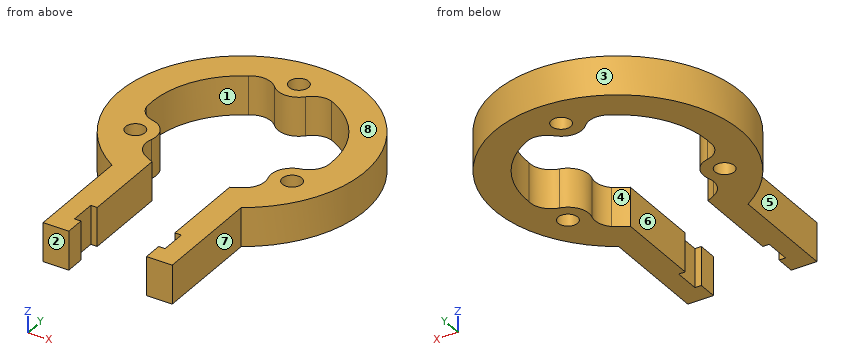
```python
from build123d import *

# Parameters (mm, degrees)
ESQUISSE1_R        = 1.5
BOSS_EXTRU_2_DEPTH = 6


with BuildPart() as part:
    # Esquisse1 → Boss.-Extru.2 (new body)
    with BuildSketch(Plane.XY):
        with BuildLine():
            Line((-6, -33.155494421), (-6, -30.155494421))
            Line((-6, -30.155494421), (-7, -30.155494421))
            Line((-7, -30.155494421), (-7, -26.155494421))
            Line((-7, -26.155494421), (-6, -26.155494421))
            Line((-6, -26.155494421), (-6, -12.649110641))
            ThreePointArc((-6, -12.649110641), (-6.653410863, -12.317959405), (-7.288606081, -11.953084179))
            ThreePointArc((-7.288606081, -11.953084179), (-8.912631465, -10.307392628), (-9.031496673, -7.998360322))
            ThreePointArc((-9.031496673, -7.998360322), (-9.309773091, -5.375), (-11.442531564, -3.822325392))
            ThreePointArc((-11.442531564, -3.822325392), (-13.054716827, -2.946828253), (-13.935938611, -1.337764944))
            ThreePointArc((-13.935938611, -1.337764944), (-12.367555464, 6.560760004), (-6.707371512, 12.288660114))
            ThreePointArc((-6.707371512, 12.288660114), (-4.47014813, 12.872261577), (-2.411034891, 11.820685714))
            ThreePointArc((-2.411034891, 11.820685714), (0, 10.75), (2.411034891, 11.820685714))
            ThreePointArc((2.411034891, 11.820685714), (3.975330286, 12.779130538), (5.80943088, 12.737759334))
            ThreePointArc((5.80943088, 12.737759334), (11.865562564, 7.430237213), (13.995977593, -0.335575935))
            ThreePointArc((13.995977593, -0.335575935), (13.382779595, -2.564868949), (11.442531564, -3.822325392))
            ThreePointArc((11.442531564, -3.822325392), (9.309773091, -5.375), (9.031496673, -7.998360322))
            ThreePointArc((9.031496673, -7.998360322), (9.079386541, -9.832302285), (8.126507731, -11.399994391))
            ThreePointArc((8.126507731, -11.399994391), (7.090812931, -12.071469338), (6, -12.649110641))
            Line((6, -12.649110641), (6, -26.155494421))
            Line((6, -26.155494421), (7, -26.155494421))
            Line((7, -26.155494421), (7, -30.155494421))
            Line((7, -30.155494421), (6, -30.155494421))
            Line((6, -30.155494421), (6, -33.155494421))
            Line((6, -33.155494421), (10, -33.155494421))
            Line((10, -33.155494421), (10, -16.155494421))
            ThreePointArc((10, -16.155494421), (0, 19), (-10, -16.155494421))
            Line((-10, -16.155494421), (-10, -33.155494421))
            Line((-10, -33.155494421), (-6, -33.155494421))
        make_face()
        with Locations((0, 14)):
            Circle(ESQUISSE1_R, mode=Mode.SUBTRACT)
        with Locations((12.124355653, -7)):
            Circle(ESQUISSE1_R, mode=Mode.SUBTRACT)
        with Locations((-12.124355653, -7)):
            Circle(ESQUISSE1_R, mode=Mode.SUBTRACT)
    extrude(amount=BOSS_EXTRU_2_DEPTH)


solid = part.part
```
The listing builds one solid part. Answer for the finished solid, in the listing's coordinates (mm). Face numbers are marked on the shaded views. A direction names the side the tool comes from. Coordinates: 2 decimals unless noted, no trailing zeros. Write each loop counter-clockwise with the first axis right and the second up, starting at its lowest first coordinate (ties: lowest second). Pieces come first, ordered by that corner, then holes. Notation, with made-up numbers: (54.25, 41) - (75.25, 41) arc R11 cw to (75.25, 49) - close; hole circle Ø4 at (2, 53). An arc over 180 degrees is marked (long way). One line per item, written item: value.
1) Each of these flat-tipped pins is pushed along its axis until it touches: pin 1 Ø2 at (x, z) = (-5, 4) entering from +Y; pin 2 Ø1.1 at (x, z) = (6.5, 1.5) entering from +Y; pin 3 Ø3.5 at (x, y) = (12.12, -7) entering from +Z; pin 4 Ø1.5 at (x, z) = (4.5, 1) entering from -Y. Where does it stop, or does it pass through?
Geometry check:
pin 1: stops at y = 18.57
pin 2: stops at y = 18.04
pin 3: stops at z = 6
pin 4: stops at y = 12.71
2) Consider line 1 along X through (y, z) = (-26.5, 2.45); line 2 along X through (y, z) = (-18.5, 5.4); line 3 along Y through (x, z) = (12.5, 5.85). Determine where each line is inside the solid, lowest interval first. Write a range as from..to.
Geometry check:
line 1: x = -10..-7, 7..10
line 2: x = -10..-6, 6..10
line 3: y = -14.31..-8.45, -5.55..-3.39, 6.3..14.31
3) Find section D-D (x = -13). Give the vertices of the cut face in (y, z).
Geometry check:
outline: (-13.86, 0) - (-8.22, 0) - (-8.22, 6) - (-13.86, 6) - close; (-5.78, 0) - (-3, 0) - (-3, 6) - (-5.78, 6) - close; (5.2, 0) - (13.86, 0) - (13.86, 6) - (5.2, 6) - close
4) Find section C-C (z = 3.5). Count the separate pieces of the cut face and the enclosed holes in it, and give its area (3 significant figures).
Geometry check:
separate pieces: 1
enclosed holes: 3
area: 611 mm2
5) For a pull along X with two mould halves and no side action, classify the marked faces 1, 2 and 3 as pulls with the +X half, pulls with the -X half, needs draft (parallel to the pull), parting line crosses it, or undercut.
Geometry check:
face 1: undercut
face 2: needs draft
face 3: parting line crosses it
6) A tool of negligible diameter and unlimited length cuts with its end or side. For the marked faces 4, 5, 6, 7 and 8, from which of +Z, -Z, +X, -X, +Y, -Y can it reach the whole face along a straight path? Write none if from no direction.
Geometry check:
face 4: +Z, -Z
face 5: +Z, -Z, -X, -Y
face 6: +Z, -Z, -Y
face 7: +Z, -Z, +X, -Y
face 8: +Z, +X, -X, +Y, -Y
7) Find section B-B (y = -22). Give the vertices of the cut face in (x, z).
Geometry check:
outline: (-10, 0) - (-6, 0) - (-6, 6) - (-10, 6) - close; (6, 0) - (10, 0) - (10, 6) - (6, 6) - close
8) Find section A-A (x = 0). Give the vertices of the cut face in (y, z), and give its area (3 significant figures).
Geometry check:
outline: (10.75, 0) - (12.5, 0) - (12.5, 6) - (10.75, 6) - close; (15.5, 0) - (19, 0) - (19, 6) - (15.5, 6) - close
area: 31.5 mm2
